Design review of the part built by this model. Coordinates are the model's own, in mm. A direction names the side the tool comes from. Coordinates: 2 decimals unless noted, no trailing zeros. Loops run counter-clockwise (first coordinate to the right, second up) from the corner with the lowest first, then second, coordinate; pieces in that order, holes last. Notation, with made-up numbers: (23, 79.5) - (46, 79.5) arc R16 ccw to (46, 85.5) - close; hole circle Ø2 at (52.25, 77.25). An arc over 180 degrees is marked (long way). One line per question, with ' | ' between items.
from build123d import *

# Parameters (mm, degrees)
RESSALTO_EXTRUS_O1_DEPTH = 5
ESBO_O1_4_W              = 106
ESBO_O1_4_H              = 21.35
ESBO_O1_4_W_2            = 21
ESBO_O1_4_H_2            = 7.5
RESSALTO_EXTRUS_O2_DEPTH = 3.5
CORTE_EXTRUS_O10_START   = -2.958856
ESBO_O3_R                = 1.25
CORTE_EXTRUS_O10_DEPTH   = 30
RESSALTO_EXTRUS_O4_DEPTH = 1


with BuildPart() as part:
    # Esboço1 → Ressalto-extrusão1 (new body)
    with BuildSketch(Plane.XY):
        Polygon((86, -2.958856089), (99, -2.958856089), (99, 18.391143911), (86, 18.391143911), (-7, 18.391143911), (-7, -2.958856089), align=None)
        Polygon((-5.5, 9.388435505), (-5.5, 16.891143911), (-3.5, 16.891143911), (17.5, 16.891143911), (87.5, 16.891143911), (97.5, 16.891143911), (97.5, -1.458856089), (87.5, -1.458856089), (-5.5, -1.458856089), align=None, mode=Mode.SUBTRACT)
    extrude(amount=RESSALTO_EXTRUS_O1_DEPTH)

    # Esboço1<4> → Ressalto-extrusão2 (add)
    with BuildSketch(Plane.XY):
        with Locations((46, 7.716143911)):
            Rectangle(ESBO_O1_4_W, ESBO_O1_4_H)
        with Locations((7, 11.141143911)):
            Rectangle(ESBO_O1_4_W_2, ESBO_O1_4_H_2, mode=Mode.SUBTRACT)
    extrude(amount=-RESSALTO_EXTRUS_O2_DEPTH)

    # Esboço3 → Corte-extrusão10 (cut)
    with BuildSketch(Plane(origin=(0, 0, 0), x_dir=(1, 0, 0), z_dir=(0, 1, 0)).offset(CORTE_EXTRUS_O10_START)):
        with Locations((2.25, 1.5)):
            Circle(ESBO_O3_R)
        with Locations((11.75, 1.5)):
            Circle(ESBO_O3_R)
    extrude(amount=CORTE_EXTRUS_O10_DEPTH, mode=Mode.SUBTRACT)

    # Esboço1<7> → Ressalto-extrusão4 (add)
    with BuildSketch(Plane.XY):
        Polygon((-3.5, 16.891143911), (-5.5, 16.891143911), (-5.5, 9.388435505), (-5.5, -1.458856089), (87.5, -1.458856089), (97.5, -1.458856089), (97.5, 16.891143911), (87.5, 16.891143911), (17.5, 16.891143911), align=None)
        Polygon((88, -0.958856089), (-5, -0.958856089), (-5, 16.391143911), (88, 16.391143911), (97, 16.391143911), (97, -0.958856089), align=None, mode=Mode.SUBTRACT)
        Polygon((97, -0.958856089), (88, -0.958856089), (-5, -0.958856089), (-5, 16.391143911), (88, 16.391143911), (97, 16.391143911), align=None)
        Polygon((17.5, 7.391143911), (17.5, 9.388435505), (17.5, 14.891143911), (-3.5, 14.891143911), (-3.5, 7.391143911), align=None, mode=Mode.SUBTRACT)
    extrude(amount=RESSALTO_EXTRUS_O4_DEPTH)


solid = part.part
Q1. To check wall thickness, follow line 1 along X through (y, z) = (5, -1.5); line 2 along Y through (x, z) = (60.5, 4.25); line 3 along X through (y, z) = (0, 4.5). State the ranges of each line that lie inside material, in increasing order.
Returned:
line 1: x = -7 to 1, 3.5 to 10.5, 13 to 99 | line 2: y = -2.96 to -1.46, 16.89 to 18.39 | line 3: x = -7 to -5.5, 97.5 to 99
Q2. Take a section at B-B (z = 3). Give the boundary of the cut face in (x, y).
Returned:
outline: (-7, -2.96) - (99, -2.96) - (99, 18.39) - (-7, 18.39) - close; hole (-5.5, -1.46) - (97.5, -1.46) - (97.5, 16.89) - (-5.5, 16.89) - close
Q3. Draft analysis for pull direction Y (two halves, no side actions). For faces 1 (the flat face through (-5.5, 8, 3)), 2 (the flat face through (45, -2.959, 1)), 3 (the flat face through (17.5, 11, -1)), 4 (the cylindrical face through (3.405, 16.617, -1.021)), state which applies: +Y half, -Y half, draft (parallel to the pull), parting line (faces both ways), or undercut.
Returned:
face 1: undercut | face 2: -Y half | face 3: undercut | face 4: draft
Q4. Take a section at C-C (x = 11.75). Give the boundary of the cut face in (y, z), plus the area to 3 significant figures.
Returned:
outline: (-2.96, -3.5) - (7.39, -3.5) - (7.39, -2.75) - (-2.96, -2.75) - close; (-2.96, -0.25) - (7.39, -0.25) - (7.39, 1) - (-1.46, 1) - (-1.46, 5) - (-2.96, 5) - close; (14.89, -3.5) - (18.39, -3.5) - (18.39, -2.75) - (14.89, -2.75) - close; (14.89, -0.25) - (18.39, -0.25) - (18.39, 5) - (16.89, 5) - (16.89, 1) - (14.89, 1) - close | area: 39.7 mm²
Q5. Tool access review of faces 5 (the flat face through (45, 8, 1)), 6 (the flat face through (7, 14.891, -1)), 7 (the flat face through (45, 8, -3.5)): name each direction out of +Z, -Z, +X, -X, +Y, -Y from which nothing blocks a thin tool from reaching the whole face with its end or side.
Returned:
face 5: +Z | face 6: +Z, -Z | face 7: -Z, +X, -X, +Y, -Y
Q6. Take a section at A-A (y = 10.25). Give the boundary of the cut face in (x, z).
Returned:
outline: (-7, -3.5) - (-3.5, -3.5) - (-3.5, 1) - (-5.5, 1) - (-5.5, 5) - (-7, 5) - close; (17.5, -3.5) - (99, -3.5) - (99, 5) - (97.5, 5) - (97.5, 1) - (17.5, 1) - close
Q7. Take a section at D-D (y = 2.25). Give the boundary of the cut face in (x, z).
Returned:
outline: (-7, -3.5) - (99, -3.5) - (99, 5) - (97.5, 5) - (97.5, 1) - (-5.5, 1) - (-5.5, 5) - (-7, 5) - close; hole circle Ø2.5 at (2.25, -1.5); hole circle Ø2.5 at (11.75, -1.5)
Q8. For pin 1 (2 mm diameter, centred on x = 13.5, y = 0, fed in from +Z), flat-tipped, find the tip position at first contact; note if it passes through.
Returned:
pin 1: stops at z = 1
